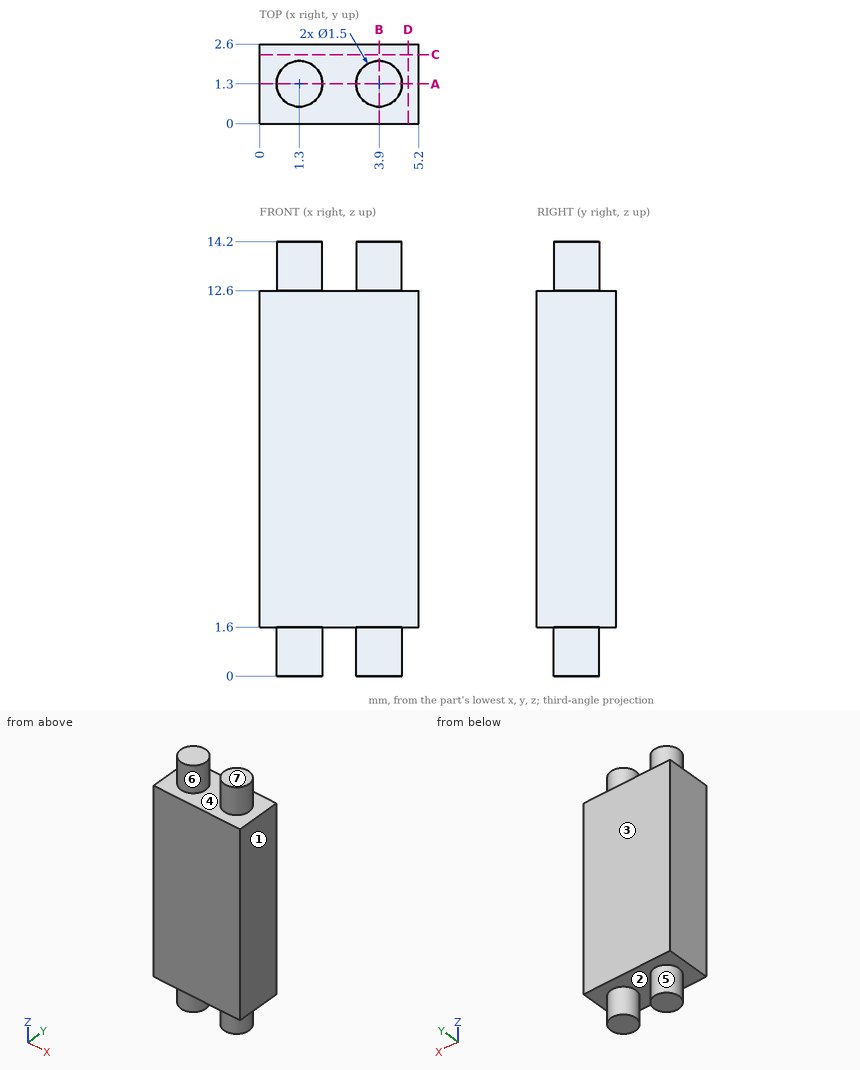
Print and shaded views of the part. All mm, measured from the part's lowest x, y and z. A direction names the side the tool comes from. Give positions to 0.01 mm unless a question says otherwise; leave off trailing zeros. Write each loop counter-clockwise with the first axis right and the second up, starting at its lowest first coordinate (ties: lowest second). Pieces come first, ordered by that corner, then holes. Notation, with made-up numbers: (77.5, 26) -> (98.5, 26) arc R26 ccw to (98.5, 61) -> close; hole circle Ø9 at (-8, 19.25). An arc over 180 degrees is marked (long way). Write item = value, one per line.
(1) Probe line 1 along Z through (x, y) = (2.95, 1.8); line 2 along X through (y, z) = (0.8, 1.25). List the from-to ranges inside material, lowest first.
Determined:
line_1 = 1.6 to 12.6
line_2 = 0.74 to 1.86, 3.34 to 4.46
(2) Slice it at C-C, the plane y = 2.25. Give the cut face in (x, z), then the cut area to 3 significant figures.
Determined:
outline = (0, 1.6) -> (5.2, 1.6) -> (5.2, 12.6) -> (0, 12.6) -> close
area = 57.2 mm2
(3) Slice it at A-A, the plane y = 1.3. Give the cut face in (x, z), then the cut area to 3 significant figures.
Determined:
outline = (0, 1.6) -> (0.55, 1.6) -> (0.55, 0) -> (2.05, 0) -> (2.05, 1.6) -> (3.15, 1.6) -> (3.15, 0) -> (4.65, 0) -> (4.65, 1.6) -> (5.2, 1.6) -> (5.2, 12.6) -> (4.65, 12.6) -> (4.65, 14.2) -> (3.15, 14.2) -> (3.15, 12.6) -> (2.05, 12.6) -> (2.05, 14.2) -> (0.55, 14.2) -> (0.55, 12.6) -> (0, 12.6) -> close
area = 66.8 mm2
(4) Slice it at B-B, the plane x = 3.9. Give the cut face in (y, z), then the cut area to 3 significant figures.
Determined:
outline = (0, 1.6) -> (0.55, 1.6) -> (0.55, 0) -> (2.05, 0) -> (2.05, 1.6) -> (2.6, 1.6) -> (2.6, 12.6) -> (2.05, 12.6) -> (2.05, 14.2) -> (0.55, 14.2) -> (0.55, 12.6) -> (0, 12.6) -> close
area = 33.4 mm2
(5) Slice it at D-D, the plane x = 4.85. Give the cut face in (y, z), then the cut area to 3 significant figures.
Determined:
outline = (0, 1.6) -> (2.6, 1.6) -> (2.6, 12.6) -> (0, 12.6) -> close
area = 28.6 mm2
(6) Mould opens along X. For the marked faces 1, 2, 3 and 4 say: released by +X, released by -X, zero draft, split by the parting line, or undercut.
Determined:
face_1 = released by +X
face_2 = undercut
face_3 = zero draft
face_4 = undercut
(7) Tool access for the marked faces 5, 6 and 7: list every direction of +Z, -Z, +X, -X, +Y, -Y with a clear straight run to the whole face (end or side of a thin tool).
Determined:
face_5 = -Z
face_6 = +Z
face_7 = +Z, +X, -X, +Y, -Y
